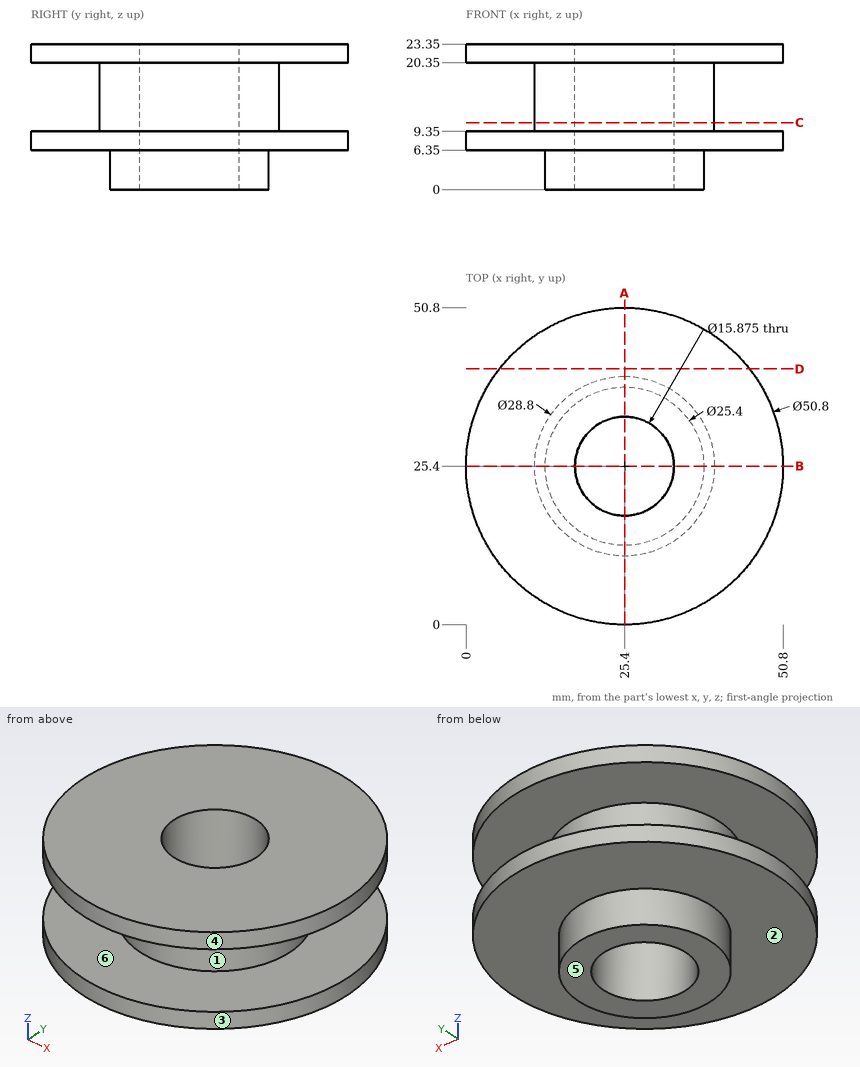
Part print with two shaded views. Sizes in mm from the minimum x, y, z corner. A direction names the side the tool comes from. Coordinates: 2 decimals unless noted, no trailing zeros. Write each loop counter-clockwise with the first axis right and the second up, starting at its lowest first coordinate (ties: lowest second). Pieces come first, ordered by that corner, then holes.
1. Drill centre lines: probe 1 along Z at (x, y) = (47.5, 25.5); probe 2 along X at (y, z) = (25.4, 13.25); probe 3 along X at (y, z) = (25.4, 6.25). Where is each one in solid material? Low to high.
Answer block:
probe 1: z = 6.35 to 9.35, 20.35 to 23.35
probe 2: x = 11 to 17.46, 33.34 to 39.8
probe 3: x = 12.7 to 17.46, 33.34 to 38.1
2. 3-axis set-ups, long thin cutter, end or side, ignore diameter. For the marked faces 1, 2 and 3: which of +Z, -Z, +X, -X, +Y, -Y reach the whole face in a straight line?
Answer block:
face 1: none
face 2: -Z
face 3: +Z, -Z
3. Band-saw the part on A-A, the plane x = 25.4. Give the cut face in (y, z), and give its area (3 significant figures).
Answer block:
outline: (0, 6.35) - (12.7, 6.35) - (12.7, 0) - (17.46, 0) - (17.46, 23.35) - (0, 23.35) - (0, 20.35) - (11, 20.35) - (11, 9.35) - (0, 9.35) - close; (33.34, 0) - (38.1, 0) - (38.1, 6.35) - (50.8, 6.35) - (50.8, 9.35) - (39.8, 9.35) - (39.8, 20.35) - (50.8, 20.35) - (50.8, 23.35) - (33.34, 23.35) - close
area: 412 mm2
4. Pull direction Z, two halves, no side cores. Call the marked faces 4, 5 and 6: released by +Z, released by -Z, zero draft, split by the parting line, or undercut.
Answer block:
face 4: zero draft
face 5: released by -Z
face 6: undercut
5. Band-saw the part on D-D, the plane y = 41. Give the cut face in (x, z).
Answer block:
outline: (5.36, 6.35) - (45.44, 6.35) - (45.44, 9.35) - (5.36, 9.35) - close; (5.36, 20.35) - (45.44, 20.35) - (45.44, 23.35) - (5.36, 23.35) - close
6. Band-saw the part on C-C, the plane z = 10.75. Give the cut face in (x, y) (1 decimal).
Answer block:
outline: circle Ø28.8 at (25.4, 25.4); hole circle Ø15.9 at (25.4, 25.4)
7. Drop flat-ended pins along their axis: pin 1 (4 mm diameter, centred on x = 30, z = 5, fed in from -Y); pin 2 (1 mm diameter, centred on y = 20.5, z = 5.5, fed in from +X); pin 3 (10 mm diameter, centred on y = 5, z = 4, fed in from +X); pin 4 (6 mm diameter, centred on x = 44, z = 3, fed in from -Y). Give the stop position or say it passes through.
Answer block:
pin 1: stops at y = 0.19
pin 2: stops at x = 37.31
pin 3: stops at x = 45.14
pin 4: passes through
